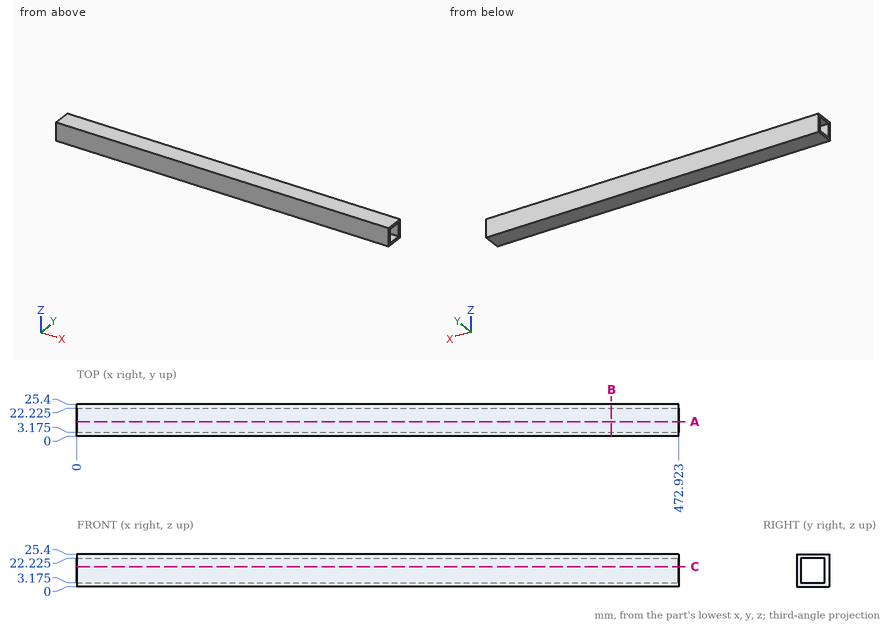
Study the drawing (mm; zero at the part's minimum x, y, z) and answer. Coordinates: 2 decimals unless noted, no trailing zeros. Write each loop counter-clockwise with the first axis right and the second up, starting at its lowest first coordinate (ties: lowest second). Pieces come first, ordered by that corner, then holes. Notation, with made-up numbers: M 36,30 L 67,30 A6 ccw 67,40 Z; hole C 37,5.25 d3. An arc over 180 degrees is marked long. Use a Markdown table: item, result. Add a question column.
1. Given P1, Ø6, axis at x = 140.5, z = 15, coming from the -Y side; P2, Ø12, axis at y = 13, z = 15.5, coming from the +X side, each flat-ended and moving along its own axis, determine where each tip first touches the part or whether it passes through.
2. Section B-B (x = 420) is taken. Give the vertices of the cut face in (y, z) (1 decimal), plus the area to 3 significant figures.
3. Section A-A (y = 11.5) is taken. Give the vertices of the cut face in (x, z) (1 decimal), plus the area to 3 significant figures.
4. A straight line is drawn through the part: line 1 along Y through (x, z) = (275, 3.5) (1 decimal). Find the intervals that lie inside material, in ascending order. Write a range as [from, to].
Data:
| question | item | result |
|---|---|---|
| 1 | P1 | stops at y = 0 |
| 1 | P2 | passes through |
| 2 | outline | M 0,0 L 25.4,0 L 25.4,25.4 L 0,25.4 Z; hole M 3.2,3.2 L 22.2,3.2 L 22.2,22.2 L 3.2,22.2 Z |
| 2 | area | 282 mm2 |
| 3 | outline | M 0,0 L 472.9,0 L 472.9,3.2 L 0,3.2 Z; M 0,22.2 L 472.9,22.2 L 472.9,25.4 L 0,25.4 Z |
| 3 | area | 3,000 mm2 |
| 4 | line 1 | y = [0, 3.2], [22.2, 25.4] |
